CAD build for the part. Positions are in the model's coordinates, mm. A direction names the side the tool comes from. Round coordinates to 2 decimals unless told otherwise and drop trailing zeros. Write each loop counter-clockwise with the first axis right and the second up, starting at its lowest first coordinate (ties: lowest second). Pieces come first, ordered by that corner, then holes. Notation, with made-up numbers: (40.25, 78.25) - (99.25, 78.25) arc R33 ccw to (99.25, 115.25) - close; hole circle Ø7 at (-30, 11). An arc over 180 degrees is marked (long way). Answer in a Markdown table with one row per item.
Autodesk Inventor part; units mm, degrees
ref_plane "YZ Plane" through (0, 0, 0) normal (1, 0, 0) x (0, 1, 0)
ref_plane "XZ Plane" through (0, 0, 0) normal (0, 1, 0) x (-1, 0, 0)
ref_plane "XY Plane" through (0, 0, 0) normal (0, 0, 1) x (1, 0, 0)
sketch "Sketch2" plane through (0, 0, 0) normal (0, 0, 1) x (1, 0, 0)
  line L0 (-53.825, 22.5) -> (53.825, 22.5)
  line L1 (53.825, 22.5) -> (53.825, -22.5)
  line L2 (53.825, -22.5) -> (-53.825, -22.5)
  line L3 (-53.825, -22.5) -> (-53.825, 22.5)
  line L4 (-48.25, 20.5) -> (48.25, 20.5)
  line L5 (48.25, -20.5) -> (-48.25, -20.5)
  line L6 (-50.25, 19.8997) -> (-50.25, -18.4997)
  line L7 (50.25, 19.3484) -> (50.25, -18.4997)
  line L8 (48.25, 14.7) -> (50.25, 14.7)
  line L9 (-50.25, 14.7) -> (-48.25, 14.7)
  line L10 (-50.25, -15.3) -> (-48.25, -15.3)
  line L11 (48.25, -15.3) -> (50.25, -15.3)
  line L12 (49.25, 14.7) -> (49.25, -15.3) construction
  line L13 (49.25, -0.3) -> (-49.8494, -0.3) construction
  line L14 (48.25, -1.3) -> (50.25, -1.3)
  line L15 (50.25, 0.7) -> (48.25, 0.7)
  line L16 (-48.25, 0.7) -> (-50.25, 0.7)
  line L17 (-48.25, -1.3) -> (-50.25, -1.3)
  line L18 (-50.25, 2.2) -> (-48.25, 2.2)
  line L19 (48.25, 2.2) -> (50.25, 2.2)
  line L20 (-50.25, -2.8) -> (-48.25, -2.8)
  line L21 (48.25, -2.8) -> (50.25, -2.8)
  line L22 (-48.25, 4.2) -> (-50.25, 4.2)
  line L23 (48.25, 4.2) -> (50.25, 4.2)
  line L24 (50.25, -4.8) -> (48.25, -4.8)
  line L25 (-48.25, -4.8) -> (-50.25, -4.8)
  line L26 (48.25, -1.3) -> (48.25, -2.8)
  line L27 (48.25, 2.2) -> (48.25, 0.7)
  line L28 (-48.25, -2.8) -> (-48.25, -1.3)
  line L29 (-48.25, 0.7) -> (-48.25, 2.2)
  line L30 (-48.25, -6.3) -> (-50.25, -6.3)
  line L31 (48.25, -6.3) -> (50.25, -6.3)
  line L32 (48.25, -8.3) -> (50.25, -8.3)
  line L33 (-48.25, -8.3) -> (-50.25, -8.3)
  line L34 (-50.25, -9.8) -> (-48.25, -9.8)
  line L35 (48.25, -9.8) -> (50.25, -9.8)
  line L36 (50.25, -11.8) -> (48.25, -11.8)
  line L37 (-48.25, -11.8) -> (-50.25, -11.8)
  line L38 (-50.25, -13.3) -> (-48.25, -13.3)
  line L39 (48.25, -13.3) -> (50.25, -13.3)
  line L40 (50.25, 5.7) -> (48.25, 5.7)
  line L41 (-48.25, 5.7) -> (-50.25, 5.7)
  line L42 (-50.25, 7.7) -> (-48.25, 7.7)
  line L43 (48.25, 7.7) -> (50.25, 7.7)
  line L44 (50.25, 9.2) -> (48.25, 9.2)
  line L45 (-48.25, 9.2) -> (-50.25, 9.2)
  line L46 (-50.25, 11.2) -> (-48.25, 11.2)
  line L47 (48.25, 11.2) -> (50.25, 11.2)
  line L48 (50.25, 12.7) -> (48.25, 12.7)
  line L49 (-48.25, 12.7) -> (-50.25, 12.7)
  line L50 (48.25, -4.8) -> (48.25, -6.3)
  line L51 (48.25, -8.3) -> (48.25, -9.8)
  line L52 (48.25, -11.8) -> (48.25, -13.3)
  line L53 (48.25, -15.3) -> (48.25, -20.5)
  line L54 (48.25, 5.7) -> (48.25, 4.2)
  line L55 (48.25, 9.2) -> (48.25, 7.7)
  line L56 (48.25, 20.5) -> (48.25, 14.7)
  line L57 (48.25, 12.7) -> (48.25, 11.2)
  line L58 (-48.25, -20.5) -> (-48.25, -15.3)
  line L59 (-48.25, -13.3) -> (-48.25, -11.8)
  line L60 (-48.25, -9.8) -> (-48.25, -8.3)
  line L61 (-48.25, -6.3) -> (-48.25, -4.8)
  line L62 (-48.25, 4.2) -> (-48.25, 5.7)
  line L63 (-48.25, 7.7) -> (-48.25, 9.2)
  line L64 (-48.25, 11.2) -> (-48.25, 12.7)
  line L65 (-48.25, 14.7) -> (-48.25, 20.5)
  point P0 (0, 0)
  dimension "d0" = 107.65
  dimension "d1" = 53.825
  dimension "d2" = 45
  dimension "d3" = 22.5
  dimension "d4" = 96.5
  dimension "d6" = 20.5
  dimension "d7" = 20.5
  dimension "d8" = 50.25
  dimension "d9" = 50.25
  dimension "d10" = 5.8
  dimension "d11" = 5.2
  dimension "d12" = 2
  dimension "d13" = 1
  dimension "d14" = 5
  dimension "d15" = 2.5
  dimension "d16" = 2
  dimension "d17" = 5
  dimension "d18" = 9
  dimension "d19" = 4.5
  dimension "d20" = 12
  dimension "d21" = 6
  dimension "d22" = 16
  dimension "d23" = 8
  dimension "d24" = 19
  dimension "d25" = 9.5
  dimension "d26" = 23
  dimension "d27" = 11.5
  dimension "d28" = 26
  dimension "d29" = 13
extrude "Extrusion1" add sketch "Sketch2" along normal blind 80.5 contours L0 L1 L2 L3 | L49 L64 L46 L6 | L7 L47 L57 L48 | L45 L63 L42 L6 | L7 L43 L55 L44 | L41 L62 L22 L6 | L7 L23 L54 L40 | L18 L29 L16 L6 | L7 L15 L27 L19 | L17 L28 L20 L6 | L7 L21 L26 L14 | L25 L61 L30 L6 | L7 L31 L50 L24 | L33 L60 L34 L6 | L7 L35 L51 L32 | L37 L59 L38 L6 | L7 L39 L52 L36
sketch "Sketch3" plane through (0, 0, 80.5) normal (0, 0, 1) x (1, 0, 0)
  circle A0 centre (48.25, -19.2) radius 1.4223
  circle A1 centre (48.25, 17.3) radius 1.3597
  point P0 (0, 0)
  dimension "d32" = 19.2
  dimension "d33" = 17.3
  dimension "d34" = 48.25
  dimension "d35" = 48.25
extrude "Extrusion2" cut sketch "Sketch3" against normal through all
mirror "Mirror1" about plane through (0, 0, 0) normal (1, 0, 0) of "Extrusion2"
properties part number "40mm_Case"
Q1. Flat gauge pin, fed straight in: pin 1 (12 mm diameter, centred on x = 29.5, y = -16.5, fed in from +Z). Where does the tip first touch, or does it go through?
Computed:
| item | result |
|---|---|
| pin 1 | stops at z = 80.5 |
Q2. Saw through at B-B on y = -19.2. List the corners of the cut face in (x, z) (3 decimals).
Computed:
| item | result |
|---|---|
| outline | (-53.825, 0) - (-49.672, 0) - (-49.672, 80.5) - (-53.825, 80.5) - close; (49.672, 0) - (53.825, 0) - (53.825, 80.5) - (49.672, 80.5) - close |
Q3. Saw through at A-A on x = -13. List the corners of the cut face in (y, z), then the cut area to 3 significant figures.
Computed:
| item | result |
|---|---|
| outline | (-22.5, 0) - (-20.5, 0) - (-20.5, 80.5) - (-22.5, 80.5) - close; (20.5, 0) - (22.5, 0) - (22.5, 80.5) - (20.5, 80.5) - close |
| area | 322 mm2 |
Q4. Pull direction X, two halves, no side cores. Call faces 3 (the flat face through (1, -22.5, 40)), 4 (the flat face through (1, -20.5, 40)), 5 (the flat face through (53.825, 0, 40)), 6 (the cylindrical face through (49.634, -19.529, 40.814)): released by +X, released by -X, zero draft, split by the parting line, or undercut.
Computed:
| item | result |
|---|---|
| face 3 | zero draft |
| face 4 | undercut |
| face 5 | released by +X |
| face 6 | undercut |
Q5. 3-axis set-ups, long thin cutter, end or side, ignore diameter. For faces 1 (the flat face through (-1, 20.5, 40)), 2 (the flat face through (-53.825, 0, 40)): which of +Z, -Z, +X, -X, +Y, -Y reach the whole face in a straight line?
Computed:
| item | result |
|---|---|
| face 1 | +Z, -Z |
| face 2 | +Z, -Z, -X, +Y, -Y |
Q6. Drill centre lines: line 1 (Y direction, x = -29, z = 18.5); line 2 (X direction, y = -15.5, z = 58.5) (3 decimals); line 3 (X direction, y = 7, z = 71) (3 decimals). Where is each one in solid material? Low to high.
Computed:
| item | result |
|---|---|
| line 1 | y = -22.5 to -20.5, 20.5 to 22.5 |
| line 2 | x = -53.825 to -48.25, 48.25 to 53.825 |
| line 3 | x = -53.825 to -50.25, 50.25 to 53.825 |
